Source: CAD feature listing. Evaluate the final solid. Frame: model axes, mm. Face numbers are marked on the shaded views. A direction names the side the tool comes from. Give positions to 0.01 mm unless a question says otherwise; leave off trailing zeros. Loops run counter-clockwise (first coordinate to the right, second up) from the corner with the lowest first, then second, coordinate; pieces in that order, holes last. Notation, with made-up numbers: (15.25, -33.5) -> (64.25, -33.5) arc R23 ccw to (64.25, -6.5) -> close; hole circle Ø8 at (88.25, 82.25). An arc over 180 degrees is marked (long way). Answer as a JSON object with one key per item and string values. Group by question number.
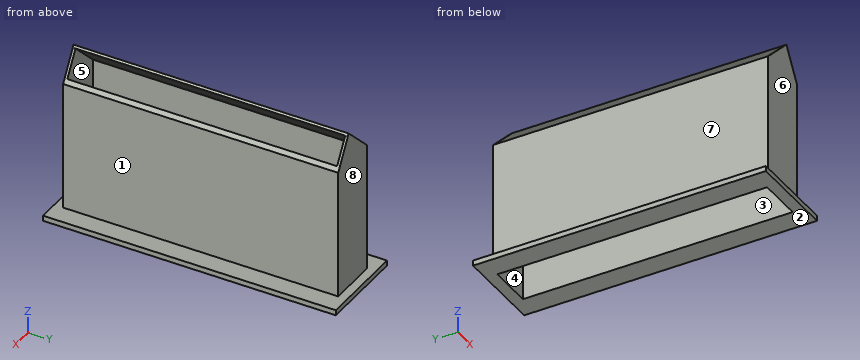
from build123d import *

# Parameters (mm, degrees)
SKETCH_1_W          = 10
SKETCH_1_H          = 33
SKETCH_1_W_2        = 5
SKETCH_1_H_2        = 30.4
EXTRUDE_1_DEPTH     = 0.6
SKETCH_2_W          = 5.6
SKETCH_2_H          = 31
SKETCH_2_W_2        = 5
SKETCH_2_H_2        = 30.4
EXTRUDE_2_DEPTH     = 18
CUT_EXTRUDE_1_DEPTH = 39.340057381
SKETCH_6_W          = 4.938455529
SKETCH_6_H          = 31
EXTRUDE_5_DEPTH     = 0.3


with BuildPart() as part:
    # 草图1 → 凸台-拉伸1 (new body)
    with BuildSketch(Plane.XY):
        with Locations((5, 16.5)):
            Rectangle(SKETCH_1_W, SKETCH_1_H)
        with Locations((5, 16.5)):
            Rectangle(SKETCH_1_W_2, SKETCH_1_H_2, mode=Mode.SUBTRACT)
    extrude(amount=EXTRUDE_1_DEPTH)

    # 草图2 → 凸台-拉伸2 (add)
    with BuildSketch(Plane.XY.offset(0.6)):
        with Locations((5, 16.5)):
            Rectangle(SKETCH_2_W, SKETCH_2_H)
        with Locations((5, 16.5)):
            Rectangle(SKETCH_2_W_2, SKETCH_2_H_2, mode=Mode.SUBTRACT)
    extrude(amount=EXTRUDE_2_DEPTH)

    # 草图5 → 切除-拉伸1 (cut, through all)
    with BuildSketch(Plane(origin=(0, 32, 0), x_dir=(1, 0, 0), z_dir=(0, 1, 0))):
        Polygon((2.2, -15.165872509), (5.748959197, -18.6), (7.8, -15.165872509), (7.8, -19.376577353), (2.2, -19.376577353), align=None)
    extrude(amount=-CUT_EXTRUDE_1_DEPTH, mode=Mode.SUBTRACT)

    # 草图6 → 凸台-拉伸5 (add)
    with BuildSketch(Plane(origin=(-6.515003899, 0, 6.732855162), x_dir=(0.7186374720968006, 0, 0.6953849176523174), z_dir=(-0.6953849176523174, 0, 0.7186374720968006))):
        with Locations((14.596349209, 16.5)):
            Rectangle(SKETCH_6_W, SKETCH_6_H)
    extrude(amount=-EXTRUDE_5_DEPTH)


solid = part.part
(1) Material intervals for line 1 (X direction, y = 11.5, z = 10.5); line 2 (Y direction, x = 4.5, z = 16.25); line 3 (Z direction, x = 1, y = 14.5), sorted ascending. Write a range as from..to.
(2) Section query B-B on z = 9.75. Return the cut outline in (x, y), plus the area to 3 significant figures.
(3) Mould query, pull axis X, two halves, no side actions, for the marked faces 1, 2, 3 and 4. Classes: pulls with the +X half, pulls with the -X half, needs draft (parallel to the pull), parting line crosses it, or undercut.
(4) Section query A-A on y = 18.5. Return the cut outline in (x, z), plus the area to 3 significant figures.
(5) Section query D-D on x = 6.5. Return the cut outline in (y, z), plus the area to 3 significant figures.
(6) First-contact query: pin 1 (1.5 mm diameter, centred on x = 3, z = 12.5, fed in from +Y); pin 2 (8 mm diameter, centred on y = 25, z = 8, fed in from +X); pin 3 (6 mm diameter, centred on x = 3, y = 28.5, fed in from +Z); pin 4 (1 mm diameter, centred on x = 8.5, z = 5.5, fed in from -Y). Flat tips, straight axial feed; report the tip coordinate or a pass-through.
(7) Section query C-C on x = 5. Return the cut outline in (y, z).
(8) Access query for the marked faces 5, 6, 7 and 8. Directions: +Z, -Z, +X, -X, +Y, -Y. A direction counts if a zero-diameter tool reaches every point of the face in a straight line with its end or side. Return the directions, or none.
Result:
{
 "1": {"line 1": "2.2..2.5, 7.5..7.8", "line 2": "1..1.3, 31.7..32", "line 3": "0..0.6"},
 "2": {"outline": "(2.2, 1) -> (7.8, 1) -> (7.8, 32) -> (2.2, 32) -> close; hole (2.5, 1.3) -> (7.5, 1.3) -> (7.5, 31.7) -> (2.5, 31.7) -> close", "area": "21.6 mm²"},
 "3": {"face 1": "pulls with the +X half", "face 2": "needs draft", "face 3": "undercut", "face 4": "undercut"},
 "4": {"outline": "(0, 0) -> (2.5, 0) -> (2.5, 15.04) -> (5.96, 18.38) -> (5.75, 18.6) -> (2.2, 15.17) -> (2.2, 0.6) -> (0, 0.6) -> close; (7.5, 0) -> (10, 0) -> (10, 0.6) -> (7.8, 0.6) -> (7.8, 15.17) -> (7.5, 15.67) -> close", "area": "13.3 mm²"},
 "5": {"outline": "(0, 0) -> (1.3, 0) -> (1.3, 17.34) -> (1, 17.34) -> (1, 0.6) -> (0, 0.6) -> close; (31.7, 0) -> (33, 0) -> (33, 0.6) -> (32, 0.6) -> (32, 17.34) -> (31.7, 17.34) -> close", "area": "11.6 mm²"},
 "6": {"pin 1": "y = 32", "pin 2": "x = 7.8", "pin 3": "z = 18.6", "pin 4": "through"},
 "7": {"outline": "(0, 0) -> (1.3, 0) -> (1.3, 17.46) -> (31.7, 17.46) -> (31.7, 0) -> (33, 0) -> (33, 0.6) -> (32, 0.6) -> (32, 17.88) -> (1, 17.88) -> (1, 0.6) -> (0, 0.6) -> close"},
 "8": {"face 5": "-Z", "face 6": "+Z, +X, -X, -Y", "face 7": "+Z, -X, +Y, -Y", "face 8": "+Z, +X, -X, +Y"}
}
